from build123d import *

# Parameters (mm, degrees)
BOSS_EXTRUDE1_DEPTH = 19.05
SKETCH3_W           = 20.32
SKETCH3_H           = 50.8
CUT_EXTRUDE1_DEPTH  = 19.05
SKETCH4_W           = 20.32
SKETCH4_H           = 50.8
CUT_EXTRUDE2_DEPTH  = 15.875
CUT_EXTRUDE3_REACH  = 110.928
SKETCH6_R           = 6.35
SKETCH6_R_2         = 1.778
CUT_EXTRUDE6_REACH  = 114.522
SKETCH9_R           = 6.35
SKETCH9_R_2         = 1.778


with BuildPart() as part:
    # Sketch1 → Boss-Extrude1 (new, symmetric)
    with BuildSketch(Plane(origin=(0, 0, 0), x_dir=(1, 0, 0), z_dir=(0, 1, 0))):
        Polygon((0, 0), (-20.32, 0), (-20.32, -50.8), (-32.385, -50.8), (-32.385, -101.6), (-29.21, -101.6), (-29.21, -53.975), (8.89, -53.975), (8.89, -101.6), (12.065, -101.6), (12.065, -50.8), (0, -50.8), align=None)
    extrude(amount=BOSS_EXTRUDE1_DEPTH, both=True)

    # Sketch3 → Cut-Extrude1 (cut)
    with BuildSketch(Plane.XZ.offset(19.05)):
        with Locations((-10.16, 25.4)):
            Rectangle(SKETCH3_W, SKETCH3_H)
    extrude(amount=-CUT_EXTRUDE1_DEPTH, mode=Mode.SUBTRACT)

    # Sketch4 → Cut-Extrude2 (cut)
    with BuildSketch(Plane(origin=(0, 19.05, 0), x_dir=(1, 0, 0), z_dir=(0, 1, 0))):
        with Locations((-10.16, -25.4)):
            Rectangle(SKETCH4_W, SKETCH4_H)
    extrude(amount=-CUT_EXTRUDE2_DEPTH, mode=Mode.SUBTRACT)

    # Sketch6 → Cut-Extrude3 (cut, up to next)
    with BuildSketch(Plane(origin=(0, 3.175, 0), x_dir=(1, 0, 0), z_dir=(0, 1, 0)), mode=Mode.PRIVATE) as cut_extrude3_sk1:
        with Locations(Location((-10.16, -10.16, 0), (0, 0, 270))):
            Circle(SKETCH6_R)
    cut_extrude3_tool1 = extrude(cut_extrude3_sk1.sketch, amount=-CUT_EXTRUDE3_REACH, mode=Mode.PRIVATE) & part.part
    # Sketch6 → Cut-Extrude3 (cut, up to next)
    with BuildSketch(Plane(origin=(0, 3.175, 0), x_dir=(1, 0, 0), z_dir=(0, 1, 0)), mode=Mode.PRIVATE) as cut_extrude3_sk2:
        with Locations(Location((-17.074797213, -17.074797213, 0), (0, 0, 270))):
            Circle(SKETCH6_R_2)
    cut_extrude3_tool2 = extrude(cut_extrude3_sk2.sketch, amount=-CUT_EXTRUDE3_REACH, mode=Mode.PRIVATE) & part.part
    # Sketch6 → Cut-Extrude3 (cut, up to next)
    with BuildSketch(Plane(origin=(0, 3.175, 0), x_dir=(1, 0, 0), z_dir=(0, 1, 0)), mode=Mode.PRIVATE) as cut_extrude3_sk3:
        with Locations(Location((-17.074797213, -3.245202787, 0), (0, 0, 270))):
            Circle(SKETCH6_R_2)
    cut_extrude3_tool3 = extrude(cut_extrude3_sk3.sketch, amount=-CUT_EXTRUDE3_REACH, mode=Mode.PRIVATE) & part.part
    # Sketch6 → Cut-Extrude3 (cut, up to next)
    with BuildSketch(Plane(origin=(0, 3.175, 0), x_dir=(1, 0, 0), z_dir=(0, 1, 0)), mode=Mode.PRIVATE) as cut_extrude3_sk4:
        with Locations(Location((-3.245202787, -3.245202787, 0), (0, 0, 270))):
            Circle(SKETCH6_R_2)
    cut_extrude3_tool4 = extrude(cut_extrude3_sk4.sketch, amount=-CUT_EXTRUDE3_REACH, mode=Mode.PRIVATE) & part.part
    # Sketch6 → Cut-Extrude3 (cut, up to next)
    with BuildSketch(Plane(origin=(0, 3.175, 0), x_dir=(1, 0, 0), z_dir=(0, 1, 0)), mode=Mode.PRIVATE) as cut_extrude3_sk5:
        with Locations(Location((-3.245202787, -17.074797213, 0), (0, 0, 270))):
            Circle(SKETCH6_R_2)
    cut_extrude3_tool5 = extrude(cut_extrude3_sk5.sketch, amount=-CUT_EXTRUDE3_REACH, mode=Mode.PRIVATE) & part.part
    add(cut_extrude3_tool1.solids().sort_by_distance((-10.16, 3.175, 10.16))[0], mode=Mode.SUBTRACT)
    add(cut_extrude3_tool2.solids().sort_by_distance((-17.074797, 3.175, 17.074797))[0], mode=Mode.SUBTRACT)
    add(cut_extrude3_tool3.solids().sort_by_distance((-17.074797, 3.175, 3.245203))[0], mode=Mode.SUBTRACT)
    add(cut_extrude3_tool4.solids().sort_by_distance((-3.245203, 3.175, 3.245203))[0], mode=Mode.SUBTRACT)
    add(cut_extrude3_tool5.solids().sort_by_distance((-3.245203, 3.175, 17.074797))[0], mode=Mode.SUBTRACT)

    # Cut-Extrude6: up to this face of the body (flat: up to its plane)
    cut_extrude6_end = Plane(part.part.faces().sort_by_distance((-32.385, 0, 76.2))[0])
    # Sketch9 → Cut-Extrude6 (cut, up to the picked face)
    with BuildSketch(Plane(origin=(12.065, 0, 0), x_dir=(0, 0, -1), z_dir=(1, 0, 0)), mode=Mode.PRIVATE) as cut_extrude6_sk1:
        with Locations((-88.9, 0)):
            Circle(SKETCH9_R)
    cut_extrude6_tool1 = split(extrude(cut_extrude6_sk1.sketch, amount=-CUT_EXTRUDE6_REACH, mode=Mode.PRIVATE), bisect_by=cut_extrude6_end, keep=Keep.BOTH, mode=Mode.PRIVATE)
    # Sketch9 → Cut-Extrude6 (cut, up to the picked face)
    with BuildSketch(Plane(origin=(12.065, 0, 0), x_dir=(0, 0, -1), z_dir=(1, 0, 0)), mode=Mode.PRIVATE) as cut_extrude6_sk2:
        with Locations((-95.814797213, 6.914797213)):
            Circle(SKETCH9_R_2)
    cut_extrude6_tool2 = split(extrude(cut_extrude6_sk2.sketch, amount=-CUT_EXTRUDE6_REACH, mode=Mode.PRIVATE), bisect_by=cut_extrude6_end, keep=Keep.BOTH, mode=Mode.PRIVATE)
    # Sketch9 → Cut-Extrude6 (cut, up to the picked face)
    with BuildSketch(Plane(origin=(12.065, 0, 0), x_dir=(0, 0, -1), z_dir=(1, 0, 0)), mode=Mode.PRIVATE) as cut_extrude6_sk3:
        with Locations((-81.985202787, 6.914797213)):
            Circle(SKETCH9_R_2)
    cut_extrude6_tool3 = split(extrude(cut_extrude6_sk3.sketch, amount=-CUT_EXTRUDE6_REACH, mode=Mode.PRIVATE), bisect_by=cut_extrude6_end, keep=Keep.BOTH, mode=Mode.PRIVATE)
    # Sketch9 → Cut-Extrude6 (cut, up to the picked face)
    with BuildSketch(Plane(origin=(12.065, 0, 0), x_dir=(0, 0, -1), z_dir=(1, 0, 0)), mode=Mode.PRIVATE) as cut_extrude6_sk4:
        with Locations((-81.985202787, -6.914797213)):
            Circle(SKETCH9_R_2)
    cut_extrude6_tool4 = split(extrude(cut_extrude6_sk4.sketch, amount=-CUT_EXTRUDE6_REACH, mode=Mode.PRIVATE), bisect_by=cut_extrude6_end, keep=Keep.BOTH, mode=Mode.PRIVATE)
    # Sketch9 → Cut-Extrude6 (cut, up to the picked face)
    with BuildSketch(Plane(origin=(12.065, 0, 0), x_dir=(0, 0, -1), z_dir=(1, 0, 0)), mode=Mode.PRIVATE) as cut_extrude6_sk5:
        with Locations((-95.814797213, -6.914797213)):
            Circle(SKETCH9_R_2)
    cut_extrude6_tool5 = split(extrude(cut_extrude6_sk5.sketch, amount=-CUT_EXTRUDE6_REACH, mode=Mode.PRIVATE), bisect_by=cut_extrude6_end, keep=Keep.BOTH, mode=Mode.PRIVATE)
    add(cut_extrude6_tool1.solids().sort_by(Axis((12.065, 0, 88.9), (-1, 0, 0)))[0], mode=Mode.SUBTRACT)
    add(cut_extrude6_tool2.solids().sort_by(Axis((12.065, 6.914797, 95.814797), (-1, 0, 0)))[0], mode=Mode.SUBTRACT)
    add(cut_extrude6_tool3.solids().sort_by(Axis((12.065, 6.914797, 81.985203), (-1, 0, 0)))[0], mode=Mode.SUBTRACT)
    add(cut_extrude6_tool4.solids().sort_by(Axis((12.065, -6.914797, 81.985203), (-1, 0, 0)))[0], mode=Mode.SUBTRACT)
    add(cut_extrude6_tool5.solids().sort_by(Axis((12.065, -6.914797, 95.814797), (-1, 0, 0)))[0], mode=Mode.SUBTRACT)


solid = part.part
Source: CAD feature listing. Evaluate the final solid. Frame: model axes, mm. A direction names the side the tool comes from. Round coordinates to 2 decimals unless told otherwise and drop trailing zeros. Loops run counter-clockwise (first coordinate to the right, second up) from the corner with the lowest first, then second, coordinate; pieces in that order, holes last. Notation, with made-up numbers: M 89,15.25 L 94,15.25 A13 ccw 94,40.25 Z; hole C -26.75,48 d4. An arc over 180 degrees is marked long. Answer as CSV lines item,"result".
Q1. Cut plane D-D (z = 88.9). Return the cut outline in (x, y) (3 decimals), plus the area to 3 significant figures.
Verdict:
outline,"M -32.385,-19.05 L -29.21,-19.05 L -29.21,-6.35 L -32.385,-6.35 Z; M -32.385,6.35 L -29.21,6.35 L -29.21,19.05 L -32.385,19.05 Z; M 8.89,-19.05 L 12.065,-19.05 L 12.065,-6.35 L 8.89,-6.35 Z; M 8.89,6.35 L 12.065,6.35 L 12.065,19.05 L 8.89,19.05 Z"
area,"161 mm^2"
Q2. Line query: line 1 along Z through (x, y) = (-17, 0.5) (3 decimals); line 2 along X through (y, z) = (-11, 69) (3 decimals); line 3 along Z through (x, y) = (10, 10). Output: solid intervals per line, ascending.
Verdict:
line 1,"z = 0 to 1.469, 5.022 to 15.298, 18.851 to 53.975"
line 2,"x = -32.385 to -29.21, 8.89 to 12.065"
line 3,"z = 50.8 to 101.6"
Q3. Contact query for flat-ended pins moving along their axis: pin 1 (12 mm diameter, centred on y = -2.5, z = 21, fed in from +X); pin 2 (4.5 mm diameter, centred on x = -17.07, z = 3.25, fed in from +Y) (3 decimals); pin 3 (2 mm diameter, centred on x = -19, y = 6, fed in from -Z); pin 4 (11.5 mm diameter, centred on x = -10.16, z = 10.16, fed in from -Y). Output: stop coordinate, or through.
Verdict:
pin 1,"stops at x = 0"
pin 2,"stops at y = 3.175"
pin 3,"stops at z = 50.8"
pin 4,"passes through"
Q4. Cut plane C-C (y = 1.5). Return the cut outline in (x, z) (3 decimals).
Verdict:
outline,"M -32.385,50.8 L -20.32,50.8 L -20.32,0 L 0,0 L 0,50.8 L 12.065,50.8 L 12.065,82.73 L 8.89,82.73 L 8.89,53.975 L -29.21,53.975 L -29.21,82.73 L -32.385,82.73 Z; M -32.385,95.07 L -29.21,95.07 L -29.21,101.6 L -32.385,101.6 Z; M 8.89,95.07 L 12.065,95.07 L 12.065,101.6 L 8.89,101.6 Z; hole C -17.075,3.245 d3.556; hole C -17.075,17.075 d3.556; hole C -10.16,10.16 d12.7; hole C -3.245,3.245 d3.556; hole C -3.245,17.075 d3.556"
Q5. Reachability of faces 4 (the face through (8.89, 0, 77)), 5 (the face through (-20.32, 2, 25)), 6 (the face through (-10, 3.175, 25)) from +Z, -Z, +X, -X, +Y, -Y: full face, straight path, thin tool, end or side. Return the list, or none.
Verdict:
face 4,"+Z, +Y, -Y"
face 5,"-Z, -X, +Y, -Y"
face 6,"-Z, +X, -X, +Y"
Q6. Pull-direction query (Y, two-part tool) for faces 1 (the face through (-10, 0, 26)), 2 (the face through (-15.312, 1.61, 16.843)), 3 (the face through (-30.775, 1.907, 82.843)); classes: +Y half, -Y half, draft (parallel to the pull), parting line (faces both ways), or undercut.
Verdict:
face 1,"-Y half"
face 2,"draft"
face 3,"undercut"
Q7. Cut plane A-A (x = -10.16). Return the cut outline in (y, z) (3 decimals).
Verdict:
outline,"M -19.05,50.8 L 0,50.8 L 0,16.51 L 3.175,16.51 L 3.175,50.8 L 19.05,50.8 L 19.05,53.975 L -19.05,53.975 Z; M 0,0 L 3.175,0 L 3.175,3.81 L 0,3.81 Z"
Q8. Cut plane B-B (z = 10.16). Return the cut outline in (x, y) (3 decimals), plus the area to 3 significant figures.
Verdict:
outline,"M -20.32,0 L -16.51,0 L -16.51,3.175 L -20.32,3.175 Z; M -3.81,0 L 0,0 L 0,3.175 L -3.81,3.175 Z"
area,"24.2 mm^2"
